Here's how the part is built. I have some questions about the finished solid (model axes, mm). A direction names the side the tool comes from. Give positions to 0.01 mm unless a question says otherwise; leave off trailing zeros. Loops run counter-clockwise (first coordinate to the right, second up) from the corner with the lowest first, then second, coordinate; pieces in that order, holes last. Notation, with made-up numbers: (33, -4.75) - (47, -4.75) arc R15 ccw to (47, 15.25) - close; hole circle Ø2 at (44.5, -21.75). An arc over 180 degrees is marked (long way). Return JSON: item names as keys, results as strings. Group by question number.
(1) If we section it at A-A (x = 34): Please give me the cut outline in (y, z), then the cut area to 3 significant figures.
(2) If we mould it in two halves opening along X, with no side actions, what happens to faces 1 (the flat face through (36, -15.276, 1)), 2 (the cylindrical face through (34.84, -2.6, 1.52)), 3 (the cylindrical face through (42.84, -2.6, 1.52)), 4 (the flat face through (29.377, 7, 1))? For each: released by +X, released by -X, zero draft, split by the parting line, or undercut.
(3) If we section it at D-D (x = 22): Please give me the cut outline in (y, z).
(4) For P1, Ø3.5, axis at x = 33.38, y = -2.28, coming from the +Z side; P2, Ø1.8, axis at x = 14.38, y = -12.28, coming from the -Z side; P3, Ø0.9, axis at x = 14.5, z = 2, coming from the +Y side; P4, Ø1.5, axis at y = 5.5, z = 2, coming from the -X side, each with a flat end and sliding along its axis, tell me the tip position at first contact or that it passes through.
(5) I need wall thicknesses on probe 1 along X at (y, z) = (-2.5, 0.2); probe 2 along Y at (x, z) = (-1, 1.5); probe 3 along X at (y, z) = (8.25, 2). Which ranges of each line are inside material? Lowest first, please. Write a range as [from, to].
(6) If we section it at B-B (y = -3): Please give me the cut outline in (x, z).
(7) If we section it at C-C (z = 1.55): Please give me the cut outline in (x, y) (3 decimals).
(8) On a 3-axis mill with a long thin cutter (end or side, diameter ignored), from which of +Z, -Z, +X, -X, +Y, -Y can I reach the whole of each face in a straight line? I mean faces 5 (the flat face through (14, -5, 3)), 6 (the flat face through (7, -1.526, 1)). Say none if no direction works.
Autodesk Inventor part; units mm, degrees
ref_plane "YZ Plane" through (0, 0, 0) normal (1, 0, 0) x (0, 1, 0)
ref_plane "XZ Plane" through (0, 0, 0) normal (0, 1, 0) x (-1, 0, 0)
ref_plane "XY Plane" through (0, 0, 0) normal (0, 0, 1) x (1, 0, 0)
sketch "Szkic1" plane through (0, 0, 0) normal (0, 0, 1) x (1, 0, 0)
  line L0 (-15.6232, -1.5262) -> (24.3768, -1.5262)
  line L1 (24.3768, -1.5262) -> (24.3768, -15.7762)
  line L2 (24.3768, -15.7762) -> (-15.6232, -15.7762)
  line L3 (-15.6232, -15.7762) -> (-15.6232, -1.5262)
  line L4 (24.3768, -1.5262) -> (29.3768, -1.5262)
  line L5 (29.3768, -1.5262) -> (29.3768, 10.7238)
  line L6 (29.3768, 10.7238) -> (45.3768, 10.7238)
  line L7 (45.3768, -15.2762) -> (45.3768, 10.7238)
  line L8 (45.3768, -15.2762) -> (24.3768, -15.2762)
  point P0 (0, 0)
  point P1 (-5.6232, -12.2762)
  point P2 (14.3768, -12.2762)
  point P3 (33.3768, -2.2762)
  point P4 (41.3768, -2.2762)
  dimension "d0" = 40
  dimension "d1" = 14.25
  dimension "d2" = 10
  dimension "d3" = 10
  dimension "d4" = 3.5
  dimension "d5" = 3.5
  dimension "d6" = 5
  dimension "d7" = 16
  dimension "d18" = 26
  dimension "d19" = 0.5
  dimension "d20" = 13
  dimension "d21" = 13
  dimension "d22" = 4
  dimension "d23" = 4
extrude "Wyciągnięcie proste1" add sketch "Szkic1" along normal blind 3
hole "Otwór1" at (-5.6232, -12.2762, 0) at (14.3768, -12.2762, 0) at (33.3768, -2.2762, 0) at (41.3768, -2.2762, 0) direction (0, 0, 1) diameter 3 end through all
chamfer "Faza1" distance 4 angle 45 1 edges at (-15.6232, -15.7762, 1.5)
fillet "Zaokrąglenie1" radius 2 2 edges at (-15.6232, -11.7762, 1.5) (-11.6232, -15.7762, 1.5)
fillet "Zaokrąglenie2" radius 5 4 edges at (-15.6232, -1.5262, 1.5) (29.3768, -1.5262, 1.5) (24.3768, -15.2762, 1.5) (24.3768, -15.7762, 1.5)
chamfer "Faza2" distance 0.5 angle 45 3 edges at (29.3768, 10.7238, 1.5) (45.3768, 10.7238, 1.5) (45.3768, -15.2762, 1.5)
properties part number "LC_ALU_3mm_Y_Axis_IGUS_Cable_Chain_Mount"
Values:
{
 "1": {"outline": "(-15.28, 0) - (-3.64, 0) - (-3.64, 3) - (-15.28, 3) - close; (-0.91, 0) - (10.72, 0) - (10.72, 3) - (-0.91, 3) - close", "area": "69.8 mm2"},
 "2": {"face 1": "zero draft", "face 2": "undercut", "face 3": "undercut", "face 4": "released by -X"},
 "3": {"outline": "(-15.78, 0) - (-1.53, 0) - (-1.53, 3) - (-15.78, 3) - close"},
 "4": {"P1": "z = 3", "P2": "through", "P3": "y = -1.53", "P4": "x = 29.38"},
 "5": {"probe 1": "[-13.59, 31.89], [34.86, 39.89], [42.86, 45.38]", "probe 2": "[-15.78, -1.53]", "probe 3": "[29.38, 45.38]"},
 "6": {"outline": "(-14.17, 0) - (32.06, 0) - (32.06, 3) - (-14.17, 3) - close; (34.69, 0) - (40.06, 0) - (40.06, 3) - (34.69, 3) - close; (42.69, 0) - (45.38, 0) - (45.38, 3) - (42.69, 3) - close"},
 "7": {"outline": "(-15.623, -10.948) arc R2 ccw to (-15.037, -12.362) - (-12.209, -15.19) arc R2 ccw to (-10.795, -15.776) - (23.434, -15.776) arc R5 ccw to (24.995, -15.526) arc R5 cw to (26.556, -15.276) - (44.877, -15.276) - (45.377, -14.776) - (45.377, 10.224) - (44.877, 10.724) - (29.877, 10.724) - (29.377, 10.224) - (29.377, 3.474) arc R5 cw to (24.377, -1.526) - (-10.623, -1.526) arc R5 ccw to (-15.623, -6.526) - close; hole circle Ø3 at (-5.623, -12.276); hole circle Ø3 at (14.377, -12.276); hole circle Ø3 at (33.377, -2.276); hole circle Ø3 at (41.377, -2.276)"},
 "8": {"face 5": "+Z, +X, -X, +Y, -Y", "face 6": "+Z, -Z, -X, +Y"}
}
